Design review of the part shown in the three views and the two pictorial views. Dimensions are in mm from the part's minimum x, y and z. A direction names the side the tool comes from. Give positions to 0.01 mm unless a question says otherwise; leave off trailing zeros. Order: outer loops, then holes, each group sorted by start corner. A loop starts at its lowest first (then second) coordinate and runs counter-clockwise, first axis right, second up.
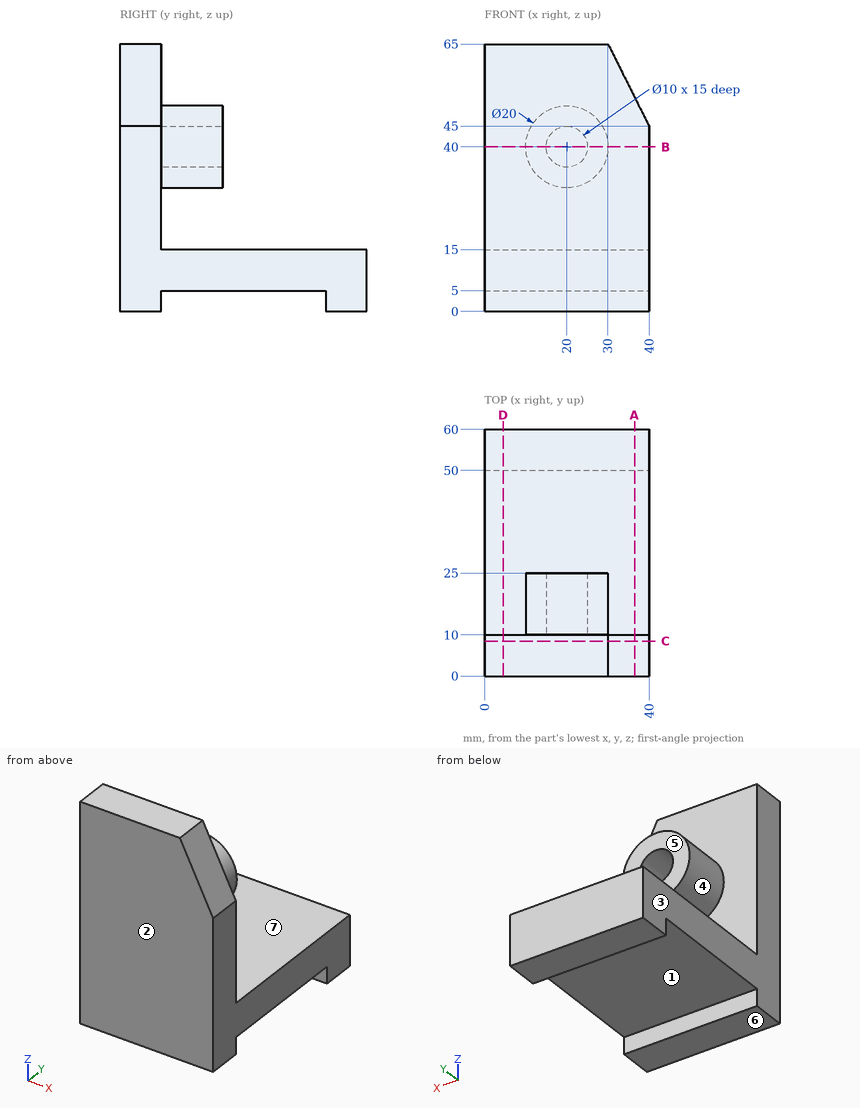
1) Draft analysis for pull direction Y (two halves, no side actions). For the marked faces 1, 2 and 3, state which applies: +Y half, -Y half, draft (parallel to the pull), parting line (faces both ways), or undercut.
Answer sheet:
face 1: undercut
face 2: -Y half
face 3: draft
2) Clearance check with flat-ended pins moving along their axes: pin 1 (5 mm diameter, centred on x = 33, y = 42.5, fed in from +Z); pin 2 (20 mm diameter, centred on x = 18, y = 34.5, fed in from -Z); pin 3 (1.5 mm diameter, centred on x = 25, z = 28.5, fed in from +Y); pin 4 (6 mm diameter, centred on x = 25.5, y = 50.5, fed in from -Z). State where each tip first meets the part, or that it passes through.
Answer sheet:
pin 1: stops at z = 15
pin 2: stops at z = 5
pin 3: stops at y = 10
pin 4: stops at z = 0
3) We need section B-B on z = 40. Give the boundary of the cut face in (x, y).
Answer sheet:
outline: (0, 0) - (40, 0) - (40, 10) - (30, 10) - (30, 25) - (25, 25) - (25, 10) - (15, 10) - (15, 25) - (10, 25) - (10, 10) - (0, 10) - close
4) We need section D-D on x = 4.5. Give the boundary of the cut face in (y, z).
Answer sheet:
outline: (0, 0) - (10, 0) - (10, 5) - (50, 5) - (50, 0) - (60, 0) - (60, 15) - (10, 15) - (10, 65) - (0, 65) - close
5) We need section A-A on x = 36.5. Give the boundary of the cut face in (y, z), then the cut area to 3 significant figures.
Answer sheet:
outline: (0, 0) - (10, 0) - (10, 5) - (50, 5) - (50, 0) - (60, 0) - (60, 15) - (10, 15) - (10, 52) - (0, 52) - close
area: 1,070 mm2
6) Tool access review of the marked faces 4, 5, 6 and 7: name each direction out of +Z, -Z, +X, -X, +Y, -Y from which nothing blocks a thin tool from reaching the whole face with its end or side.
Answer sheet:
face 4: +Y
face 5: +Z, +X, -X, +Y
face 6: -Z, +X, -X, +Y, -Y
face 7: +X, -X, +Y
7) We need section C-C on y = 8.5. Give the boundary of the cut face in (x, z).
Answer sheet:
outline: (0, 0) - (40, 0) - (40, 45) - (30, 65) - (0, 65) - close
8) To check wall thickness, follow line 1 (X direction, y = 18, z = 40); line 2 (Y direction, x = 9, z = 18); line 3 (Z direction, x = 27.5, y = 44). State the ranges of each line that lie inside material, in increasing order.
Answer sheet:
line 1: x = 10 to 15, 25 to 30
line 2: y = 0 to 10
line 3: z = 5 to 15
